Check sheet for the drawn part. Datum: minimum x, y, z corner. Units: mm. A direction names the side the tool comes from. Coordinates: 2 decimals unless noted, no trailing zeros. Loops run counter-clockwise (first coordinate to the right, second up) from the corner with the lowest first, then second, coordinate; pieces in that order, holes last. Notation, with made-up numbers: M 6,62 L 47,62 A20 cw 47,72 Z; hole C 81.5,-9 d5. An arc over 180 degrees is marked long. Use CSV: the item, a comma, the result in double quotes. Start each with the question number.
(1) Set-up check for the marked faces 1 and 2: record each of +Z, -Z, +X, -X, +Y, -Y from which the full face is reachable in a straight line by a thin tool's end or side.
(2) Section check A-A on z = 60. Record the cut outline in (x, y).
(3) Go/stop test with a flat-tipped pin: pin 1 Ø1.5 at (x, y) = (5.5, 1) entering from -Z. Record where the tip stops, or that it passes through.
(4) Section check B-B on x = 6.5. Record the cut outline in (y, z).
(5) Scan lines: line 1 (Z direction, x = 5.75, y = 5.25); line 2 (X direction, y = 3.5, z = 5.5) (1 decimal). Record each from-to range of solid material in increasing order.
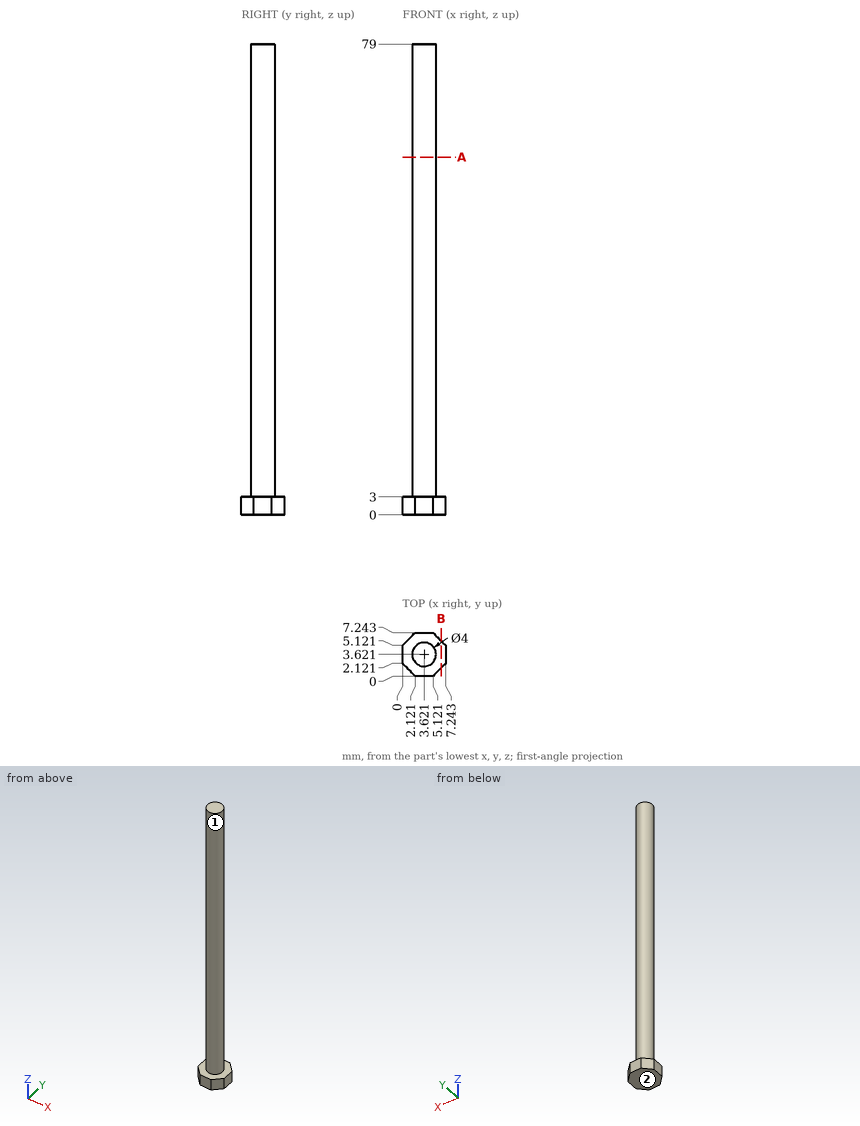
Outcome:
1,face 1,"+Z"
1,face 2,"-Z, +X, -X, +Y, -Y"
2,outline,"C 3.62,3.62 d4"
3,pin 1,"stops at z = 0"
4,outline,"M 1.38,0 L 5.86,0 L 5.86,3 L 1.38,3 Z"
5,line 1,"z = 0 to 3"
5,line 2,"x = 1.6 to 5.6"
